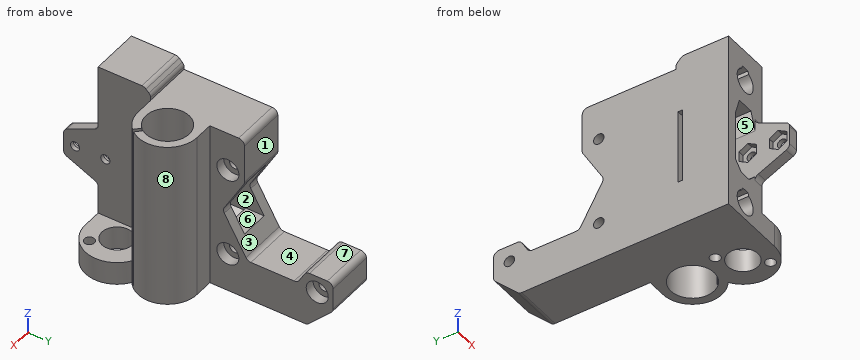
```python
from build123d import *

# Parameters (mm, degrees)
SKETCH1_R           = 1.825
SKETCH1_W           = 26
SKETCH1_H           = 1.5
BOSS_EXTRUDE1_DEPTH = 17
BOSS_EXTRUDE2_DEPTH = 58
BOSS_EXTRUDE4_DEPTH = 3.5
SKETCH9_R           = 7.5
CUT_EXTRUDE5_DEPTH  = 61
SKETCH18_R          = 1.6
CUT_EXTRUDE12_DEPTH = 5.5
CUT_EXTRUDE13_START = 1.5
CUT_EXTRUDE13_DEPTH = 3.5
FILLET1_R           = 2
SKETCH3_W           = 10
SKETCH3_H           = 20
CUT_EXTRUDE1_DEPTH  = 13
CUT_EXTRUDE2_DEPTH  = 42
SKETCH5_R           = 3.825
SKETCH5_R_2         = 9.1924e-05
CUT_EXTRUDE3_DEPTH  = 3.5
CUT_EXTRUDE4_DEPTH  = 38
SKETCH11_R          = 5.25
BOSS_EXTRUDE3_DEPTH = 8
CUT_EXTRUDE6_DEPTH  = 57
SKETCH12_R          = 1.75
CUT_EXTRUDE9_DEPTH  = 10
CUT_EXTRUDE10_DEPTH = 3
SKETCH20_R          = 4.738046486
CUT_EXTRUDE14_DEPTH = 5


with BuildPart() as part:
    # Sketch1 → Boss-Extrude1 (new body)
    with BuildSketch(Plane(origin=(50, 0, 0), x_dir=(0, 0, -1), z_dir=(1, 0, 0))):
        Polygon((-62, -12.5), (-59.799999237, -10.300000191), (-58, -10.300000191), (-58, 22.251573162), (-42.115229422, 22.251573162), (-29, 14.679491924), (-14, 23.339745962), (-14, 40.660254038), (-19.243964356, 43.68785827), (-19.243964356, 53), (-8.961172368, 53), (0, 44.038826034), (0, -28.5), (-62, -28.5), align=None)
        with Locations((-44.5, 16.5)):
            Circle(SKETCH1_R, mode=Mode.SUBTRACT)
        with Locations((-13.5, 16.5)):
            Circle(SKETCH1_R, mode=Mode.SUBTRACT)
        with Locations((-13.5, 47.5)):
            Circle(SKETCH1_R, mode=Mode.SUBTRACT)
        with Locations((-29, -11.75)):
            Rectangle(SKETCH1_W, SKETCH1_H, mode=Mode.SUBTRACT)
    extrude(amount=BOSS_EXTRUDE1_DEPTH)

    # Sketch8 → Boss-Extrude2 (add)
    with BuildSketch(Plane.XY.offset(58)):
        with BuildLine():
            ThreePointArc((73.5, -10.25), (83.75, 0), (73.5, 10.25))
            Line((73.5, 10.25), (67, 10.25))
            Line((67, 10.25), (67, -10.25))
            Line((67, -10.25), (73.5, -10.25))
        make_face()
    extrude(amount=-BOSS_EXTRUDE2_DEPTH)

    # Sketch17 → Boss-Extrude4 (add)
    with BuildSketch(Plane(origin=(67, 0, 0), x_dir=(0, 0, -1), z_dir=(1, 0, 0))):
        Polygon((-33.5, -40.5), (-39, -28.5), (-19, -28.5), (-24.5, -40.5), align=None)
    extrude(amount=-BOSS_EXTRUDE4_DEPTH)

    # Sketch9 → Cut-Extrude5 (cut)
    with BuildSketch(Plane.XY.offset(58)):
        with Locations((73.5, 0)):
            Circle(SKETCH9_R)
    extrude(amount=-CUT_EXTRUDE5_DEPTH, mode=Mode.SUBTRACT)

    # Sketch18 → Cut-Extrude12 (cut)
    with BuildSketch(Plane(origin=(67, 0, 0), x_dir=(0, 0, -1), z_dir=(1, 0, 0))):
        with Locations((-29, -36.5)):
            Circle(SKETCH18_R)
        with Locations((-29, -26)):
            Circle(SKETCH18_R)
    extrude(amount=-CUT_EXTRUDE12_DEPTH, mode=Mode.SUBTRACT)

    # Sketch19 → Cut-Extrude13 (cut)
    with BuildSketch(Plane.ZY.offset(-67).offset(CUT_EXTRUDE13_START)):
        Polygon((30.760918321, -33.45), (27.239081679, -33.45), (25.478163358, -36.5), (27.239081679, -39.55), (30.760918321, -39.55), (32.521836642, -36.5), align=None)
        Polygon((32.521836642, -26), (30.760918321, -22.95), (27.239081679, -22.95), (25.478163358, -26), (27.239081679, -29.05), (30.760918321, -29.05), align=None)
    extrude(amount=CUT_EXTRUDE13_DEPTH, mode=Mode.SUBTRACT)

    # Fillet1
    fillet1_edges = [part.edges().sort_by_distance(p)[0] for p in [
        (58.5, -12.5, 62),
        (58.5, -10.300000191, 59.799999237),
        (58.5, 22.251573162, 58),
        (58.5, 22.251573162, 42.115229422),
        (58.5, 14.679491924, 29),
        (58.5, 23.339745962, 14),
        (58.5, 40.660254038, 14),
        (58.5, 43.68785827, 19.243964356),
        (58.5, 53, 19.243964356),
        (58.5, 53, 8.961172368),
        (58.5, 44.038826034, 0),
        (65.25, -40.5, 24.5),
        (65.25, -40.5, 33.5),
        (65.25, -28.5, 39),
        (65.25, -28.5, 19),
    ]]
    fillet(fillet1_edges, radius=FILLET1_R)

    # Sketch3 → Cut-Extrude1 (cut)
    with BuildSketch(Plane(origin=(0, 22.251573162, 0), x_dir=(1, 0, 0), z_dir=(0, 1, 0))):
        with Locations((58.5, -30)):
            Rectangle(SKETCH3_W, SKETCH3_H)
    extrude(amount=-CUT_EXTRUDE1_DEPTH, mode=Mode.SUBTRACT)

    # Sketch4 → Cut-Extrude2 (cut)
    with BuildSketch(Plane.XZ.offset(28.5)):
        Polygon((53.5, 19), (56.571100235, 16), (60.5, 16), (63.5, 19.071100235), (63.5, 36), (61.454799652, 42), (55.545200348, 42), (53.5, 36), align=None)
    extrude(amount=-CUT_EXTRUDE2_DEPTH, mode=Mode.SUBTRACT)

    # Sketch5 → Cut-Extrude3 (cut)
    # profile 1 of 3: a face of its own
    with BuildSketch(Plane(origin=(67, 0, 0), x_dir=(0, 0, -1), z_dir=(1, 0, 0))):
        with Locations((-13.5, 16.5)):
            Circle(SKETCH5_R)
    # profile 2 of 3: a face of its own
    with BuildSketch(Plane(origin=(67, 0, 0), x_dir=(0, 0, -1), z_dir=(1, 0, 0))):
        with Locations((-44.5, 16.5)):
            Circle(SKETCH5_R)
    # profile 3 of 3: a face of its own
    with BuildSketch(Plane(origin=(67, 0, 0), x_dir=(0, 0, -1), z_dir=(1, 0, 0))):
        with Locations((-13.5, 47.5)):
            Circle(SKETCH5_R)
        with Locations((-13.5, 47.5)):
            Circle(SKETCH5_R_2, mode=Mode.SUBTRACT)
    extrude(amount=-CUT_EXTRUDE3_DEPTH, mode=Mode.SUBTRACT)

    # Sketch7 → Cut-Extrude4 (cut)
    with BuildSketch(Plane.XZ.offset(28.5)):
        with BuildLine():
            Line((56.751731208, 54.680921248), (57.129943038, 55.738046486))
            Line((57.129943038, 55.738046486), (59.920023802, 55.738046486))
            Line((59.920023802, 55.738046486), (60.269111237, 54.670949527))
            ThreePointArc((60.269111237, 54.670949527), (58.488447481, 46.925016376), (56.751731208, 54.680921248))
        make_face()
        with BuildLine():
            Line((56.751731208, 9.680921248), (57.129943038, 10.738046486))
            Line((57.129943038, 10.738046486), (59.920023802, 10.738046486))
            Line((59.920023802, 10.738046486), (60.269111237, 9.670949527))
            ThreePointArc((60.269111237, 9.670949527), (58.488447481, 1.925016376), (56.751731208, 9.680921248))
        make_face()
    extrude(amount=-CUT_EXTRUDE4_DEPTH, mode=Mode.SUBTRACT)

    # Sketch11 → Boss-Extrude3 (add)
    with BuildSketch(Plane(origin=(0, 0, 0), x_dir=(-1, 0, 0), z_dir=(0, 0, -1))):
        with BuildLine():
            Line((-73.5, -28.5), (-67, -28.5))
            Line((-67, -28.5), (-67, -7.732421496))
            Line((-67, -7.732421496), (-78.559091832, -7.732421496))
            ThreePointArc((-78.559091832, -7.732421496), (-84.18745441, -20.103520353), (-73.5, -28.5))
        make_face()
        with Locations(Location((-73.5, -17.5, 0), (0, 0, 90))):
            Circle(SKETCH11_R, mode=Mode.SUBTRACT)
    extrude(amount=-BOSS_EXTRUDE3_DEPTH)

    # Sketch10 → Cut-Extrude6 (cut)
    with BuildSketch(Plane.XY.offset(58)):
        Polygon((81.072283805, -7.35323434), (78.440260846, -4.840560214), (79.279772993, -3.982978679), (81.857582145, -6.443897318), align=None)
    extrude(amount=-CUT_EXTRUDE6_DEPTH, mode=Mode.SUBTRACT)

    # Sketch12 → Cut-Extrude9 (cut)
    with BuildSketch(Plane(origin=(0, 0, 0), x_dir=(-1, 0, 0), z_dir=(0, 0, -1))):
        with Locations(Location((-68.16033141, -11.542824549, 0), (0, 0, 90))):
            Circle(SKETCH12_R)
        with Locations(Location((-78.83966859, -23.457175451, 0), (0, 0, 90))):
            Circle(SKETCH12_R)
    extrude(amount=-CUT_EXTRUDE9_DEPTH, mode=Mode.SUBTRACT)

    # Sketch13 → Cut-Extrude10 (cut)
    with BuildSketch(Plane.XY.offset(8)):
        Polygon((82.389929098, -23.513303191), (80.663406893, -20.410623531), (77.113146384, -20.354495791), (75.289408081, -23.401047711), (77.015930287, -26.503727371), (80.566190795, -26.559855111), align=None)
        Polygon((67.351855423, -15.000260966), (70.750321186, -13.971703501), (71.558797173, -10.514267084), (68.968807398, -8.085388132), (65.570341635, -9.113945597), (64.761865648, -12.571382014), align=None)
    extrude(amount=CUT_EXTRUDE10_DEPTH, mode=Mode.SUBTRACT)

    # Sketch20 → Cut-Extrude14 (cut)
    with BuildSketch(Plane.XZ.offset(-9.5)):
        with Locations((58.5, 6)):
            Circle(SKETCH20_R)
        with Locations((58.5, 51)):
            Circle(SKETCH20_R)
    extrude(amount=CUT_EXTRUDE14_DEPTH, mode=Mode.SUBTRACT)


solid = part.part
```
Input: part model. Units: mm. Frame: model coordinates. Face numbers are marked on the shaded views. A direction names the side the tool comes from. Coordinates: 2 decimals unless noted, no trailing zeros. Loops run counter-clockwise (first coordinate to the right, second up) from the corner with the lowest first, then second, coordinate; pieces in that order, holes last. Notation, with made-up numbers: M 81.5,-7 L 92.5,-7 A12 ccw 92.5,8 Z; hole C 61.25,51 d5. An arc over 180 degrees is marked long. Use a Markdown table: item, result. Add a question column.
1) Draft query along Y for the marked faces 1, 2, 3 and 4. Return one class per face: +Y half, -Y half, draft (parallel to the pull), parting line (faces both ways), or undercut.
2) Section A-A, the plane y = -17.5. Return the cut outline in (x, z) (3 decimals), plus the area to 3 significant figures.
3) Section B-B, the plane x = 58.5. Give the number of separate pieces and of enclosed holes in the cut face, plus the area to 3 significant figures.
4) Set-up query: the marked faces 5, 6, 7 and 8. Return all of +Z, -Z, +X, -X, +Y, -Y with unobstructed straight access to the full face (end or side cutting, diameter ignored); none if empty.
5) Line query: L1, parallel to Z at x = 58.5, y = -7.5 (3 decimals); L2, parallel to Z at x = 58.5, y = -15 (3 decimals); L3, parallel to X at y = 5, z = 24.5. Output: solid intervals per line, ascending. Write a range as from..to.
6) Pin query (flat end, axial travel): P1, Ø10, axis at x = 80.5, z = 17.5, coming from the +Y side; P2, Ø3, axis at x = 57.5, z = 4.5, coming from the -Y side; P3, Ø3.5, axis at y = 47.5, z = 13.5, coming from the +X side; P4, Ø11, axis at x = 58.5, z = 51, coming from the +Y side. Return the tip coordinate at first contact, or that it passes through.
Answer below:
| question | item | result |
|---|---|---|
| 1 | face 1 | +Y half |
| 1 | face 2 | draft |
| 1 | face 3 | undercut |
| 1 | face 4 | undercut |
| 2 | outline | M 50,0 L 68.25,0 L 68.25,8 L 67,8 L 67,62 L 50,62 Z; M 78.75,0 L 84.5,0 L 84.5,8 L 78.75,8 Z; hole M 53.5,19 L 56.571,16 L 60.5,16 L 63.5,19.071 L 63.5,36 L 61.455,42 L 55.545,42 L 53.5,36 Z; hole M 56.752,9.681 A4.075 ccw long 60.269,9.671 L 59.92,10.738 L 57.13,10.738 Z; hole M 56.752,54.681 A4.075 ccw long 60.269,54.671 L 59.92,55.738 L 57.13,55.738 Z |
| 2 | area | 762 mm2 |
| 3 | separate pieces | 2 |
| 3 | enclosed holes | 3 |
| 3 | area | 1,480 mm2 |
| 4 | face 5 | -Y |
| 4 | face 6 | +Y, -Y |
| 4 | face 7 | +Z, +X, -X, +Y |
| 4 | face 8 | +Z, +X |
| 5 | L1 | 0..1.925, 10.738..16, 42..46.925, 55.738..58 |
| 5 | L2 | 0..1.925, 10.738..16, 42..46.925, 55.738..62 |
| 5 | L3 | 50..53.5, 63.5..67.91, 79.09..82.45 |
| 6 | P1 | y = 10.05 |
| 6 | P2 | y = 9.5 |
| 6 | P3 | through |
| 6 | P4 | y = 22.25 |
